from build123d import *

# Parameters (mm, degrees)
SKETCH1_R           = 1.6
BOSS_EXTRUDE1_DEPTH = 8
CHAMFER1_SIZE       = 1


with BuildPart() as part:
    # Sketch1 → Boss-Extrude1 (new body)
    with BuildSketch(Plane.XY):
        with BuildLine():
            Line((-0.5, 3), (60.5, 3))
            ThreePointArc((60.5, 3), (62.267766953, 2.267766953), (63, 0.5))
            Line((63, 0.5), (63, -0.5))
            ThreePointArc((63, -0.5), (62.267766953, -2.267766953), (60.5, -3))
            Line((60.5, -3), (-0.5, -3))
            ThreePointArc((-0.5, -3), (-2.267766953, -2.267766953), (-3, -0.5))
            Line((-3, -0.5), (-3, 0.5))
            ThreePointArc((-3, 0.5), (-2.267766953, 2.267766953), (-0.5, 3))
        make_face()
        Circle(SKETCH1_R, mode=Mode.SUBTRACT)
        with Locations((7.5, 0)):
            Circle(SKETCH1_R, mode=Mode.SUBTRACT)
        with Locations((15, 0)):
            Circle(SKETCH1_R, mode=Mode.SUBTRACT)
        with Locations((22.5, 0)):
            Circle(SKETCH1_R, mode=Mode.SUBTRACT)
        with Locations((30, 0)):
            Circle(SKETCH1_R, mode=Mode.SUBTRACT)
        with Locations((37.5, 0)):
            Circle(SKETCH1_R, mode=Mode.SUBTRACT)
        with Locations((45, 0)):
            Circle(SKETCH1_R, mode=Mode.SUBTRACT)
        with Locations((52.5, 0)):
            Circle(SKETCH1_R, mode=Mode.SUBTRACT)
        with Locations((60, 0)):
            Circle(SKETCH1_R, mode=Mode.SUBTRACT)
    extrude(amount=BOSS_EXTRUDE1_DEPTH)

    # Chamfer1
    chamfer1_edges = [part.edges().sort_by_distance(p)[0] for p in [
        (-1.6, 0, 0),
        (-1.6, 0, 8),
        (5.9, 0, 0),
        (5.9, 0, 8),
        (13.4, 0, 0),
        (13.4, 0, 8),
        (20.9, 0, 0),
        (20.9, 0, 8),
        (28.4, 0, 0),
        (28.4, 0, 8),
        (35.9, 0, 0),
        (35.9, 0, 8),
        (43.4, 0, 0),
        (43.4, 0, 8),
        (50.9, 0, 0),
        (50.9, 0, 8),
        (58.4, 0, 0),
        (58.4, 0, 8),
    ]]
    chamfer(chamfer1_edges, length=CHAMFER1_SIZE)


solid = part.part
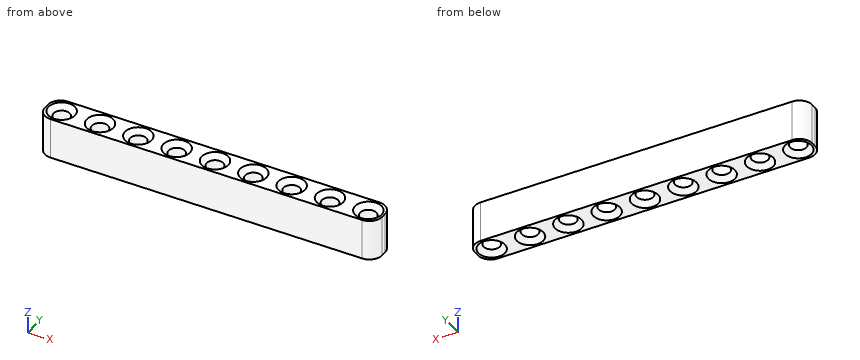
Can you work these out from the model? Positions are in its coordinate system, mm. Round coordinates to 2 decimals unless told otherwise and drop trailing zeros. Loops run counter-clockwise (first coordinate to the right, second up) from the corner with the lowest first, then second, coordinate; pieces in that order, holes last. Notation, with made-up numbers: (66.5, 84.25) - (71.5, 84.25) arc R12 cw to (71.5, 95.25) - close; hole circle Ø6 at (25, -37). An arc over 180 degrees is marked (long way). Answer in a Markdown table with one row per item. Add a question column.
Q1. I want a section at A-A on x = 45. List the corners of the cut face in (y, z) for me.
Q2. I need wall thicknesses on L1, parallel to Y at x = 52.5, z = 4.5; L2, parallel to Y at x = 7, z = 4.75; L3, parallel to Z at x = 32, y = -1.65. Which ranges of each line are inside material? Lowest first, please.
Q3. For pin 1 Ø3.5 at (x, y) = (60, 0) entering from -Z, with a flat end and sliding along its axis, tell me the tip position at first contact or that it passes through.
A:
| question | item | result |
|---|---|---|
| 1 | outline | (-3, 0) - (-2.6, 0) - (-1.6, 1) - (-1.6, 7) - (-2.6, 8) - (-3, 8) - close; (1.6, 1) - (2.6, 0) - (3, 0) - (3, 8) - (2.6, 8) - (1.6, 7) - close |
| 2 | L1 | -3 to -1.6, 1.6 to 3 |
| 2 | L2 | -3 to -1.52, 1.52 to 3 |
| 2 | L3 | 0.01 to 7.99 |
| 3 | pin 1 | z = 0.85 |
